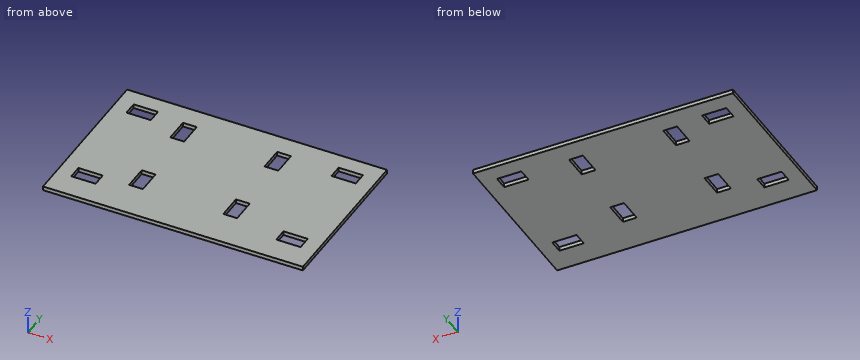
from build123d import *

# Parameters (mm, degrees)
F0_W     = 160
F0_H     = 100
F0_W_2   = 15
F0_H_2   = 8.5
F0_W_3   = 8.5
F0_H_3   = 15
F1_DEPTH = 2.5


with BuildPart() as f1:
    # F0 (on Top) → F1 (new body)
    with BuildSketch(Plane.XY):
        with Locations((-542.905006, -253.202301)):
            Rectangle(F0_W, F0_H)
        with Locations((-606.005006, -283.502301)):
            Rectangle(F0_W_2, F0_H_2, mode=Mode.SUBTRACT)
        with Locations((-577.555006, -272.702301)):
            Rectangle(F0_W_3, F0_H_3, mode=Mode.SUBTRACT)
        with Locations((-479.805006, -283.502301)):
            Rectangle(F0_W_2, F0_H_2, mode=Mode.SUBTRACT)
        with Locations((-519.555006, -272.702301)):
            Rectangle(F0_W_3, F0_H_3, mode=Mode.SUBTRACT)
        with Locations((-606.005006, -217.852301)):
            Rectangle(F0_W_2, F0_H_2, mode=Mode.SUBTRACT)
        with Locations((-577.555006, -223.702301)):
            Rectangle(F0_W_3, F0_H_3, mode=Mode.SUBTRACT)
        with Locations((-519.555006, -223.702301)):
            Rectangle(F0_W_3, F0_H_3, mode=Mode.SUBTRACT)
        with Locations((-479.805006, -217.852301)):
            Rectangle(F0_W_2, F0_H_2, mode=Mode.SUBTRACT)
    extrude(amount=F1_DEPTH)


solid = f1.part
Build history of the part. All positions in model axes, mm. Round coordinates to 2 decimals unless told otherwise and drop trailing zeros. Order: outer loops, then holes, each group sorted by start corner. A loop starts at its lowest first (then second) coordinate and runs counter-clockwise, first axis right, second up. Notation, with made-up numbers: M 27.25,37 L 46.25,37 A17 ccw 46.25,59 Z; hole C 68.5,39.5 d7. An arc over 180 degrees is marked long. Use CSV: the item, a comma, the result in double quotes. Start each with the question number.
(1) Cut at B-B on x = -482. List the corners of the cut face in (y, z), then the cut area to 4 significant figures.
(2) Cut at A-A on y = -225. List the corners of the cut face in (x, z) (3 decimals).
(3) Drill centre lines: probe 1 along X at (y, z) = (-285, 0.85) (3 decimals); probe 2 along X at (y, z) = (-266, 2.25) (3 decimals); probe 3 along Y at (x, z) = (-482, 0.6). Where is each one in solid material? Low to high.
(4) Cut at C-C on z = 0.9. State how many separate pieces and enclosed holes the cut face has, then the cut area to 3 significant figures.
Findings:
1,outline,"M -303.2,0 L -287.75,0 L -287.75,2.5 L -303.2,2.5 Z; M -279.25,0 L -222.1,0 L -222.1,2.5 L -279.25,2.5 Z; M -213.6,0 L -203.2,0 L -203.2,2.5 L -213.6,2.5 Z"
1,area,"207.5 mm^2"
2,outline,"M -622.905,0 L -581.805,0 L -581.805,2.5 L -622.905,2.5 Z; M -573.305,0 L -523.805,0 L -523.805,2.5 L -573.305,2.5 Z; M -515.305,0 L -462.905,0 L -462.905,2.5 L -515.305,2.5 Z"
3,probe 1,"x = -622.905 to -613.505, -598.505 to -487.305, -472.305 to -462.905"
3,probe 2,"x = -622.905 to -581.805, -573.305 to -523.805, -515.305 to -462.905"
3,probe 3,"y = -303.2 to -287.75, -279.25 to -222.1, -213.6 to -203.2"
4,separate pieces,"1"
4,enclosed holes,"8"
4,area,"15,000 mm^2"
